```python
from build123d import *

# Parameters (mm, degrees)
BOSS_EXTRUDE1_DEPTH      = 2.5
BOSS_EXTRUDE1_DEPTH_BACK = 2.5
SKETCH1_R                = 18.5
SKETCH1_R_2              = 12.5
SKETCH2_R                = 1.5
CUT_EXTRUDE1_DEPTH       = 10


with BuildPart() as part:
    # Sketch1 → Boss-Extrude1 (new, two sides: drawn at the far end of the back side and taken through both)
    # profile 1 of 2: a face of its own
    with BuildSketch(Plane.XY.offset(-BOSS_EXTRUDE1_DEPTH_BACK)):
        with BuildLine():
            ThreePointArc((18.5, 0), (0, -18.5), (-18.5, 0))
            Line((-18.5, 0), (-18.5, -18.75))
            Line((-18.5, -18.75), (18.5, -18.75))
            Line((18.5, -18.75), (18.5, 0))
        make_face()
    # profile 2 of 2: a face of its own
    with BuildSketch(Plane.XY.offset(-BOSS_EXTRUDE1_DEPTH_BACK)):
        Circle(SKETCH1_R)
        Circle(SKETCH1_R_2, mode=Mode.SUBTRACT)
    extrude(amount=BOSS_EXTRUDE1_DEPTH + BOSS_EXTRUDE1_DEPTH_BACK)

    # Sketch2 → Cut-Extrude1 (cut)
    with BuildSketch(Plane.XZ.offset(18.75)):
        with Locations(Location((-16, 0, 0), (0, 0, 270))):
            Circle(SKETCH2_R)
    cut_extrude1 = extrude(amount=-CUT_EXTRUDE1_DEPTH, mode=Mode.SUBTRACT)

    # Mirror1: Cut-Extrude1 across plane
    add(cut_extrude1.mirror(Plane(origin=(0, 0, 0), x_dir=(0, 0, 1), z_dir=(1, 0, 0))), mode=Mode.SUBTRACT)


solid = part.part
```
Here's how the part is built. I have some questions about the finished solid (model axes, mm). A direction names the side the tool comes from. Round coordinates to 2 decimals unless told otherwise and drop trailing zeros. Write each loop counter-clockwise with the first axis right and the second up, starting at its lowest first coordinate (ties: lowest second). Pieces come first, ordered by that corner, then holes. Notation, with made-up numbers: M 0,-11.5 L 40,-11.5 A26 cw 40,3.5 Z; hole C -9,-0.75 d8. An arc over 180 degrees is marked long. Answer as CSV lines item,"result". Start each with the question number.
1. Suppose I cut it at D-D on y = -14. Write out the boundary of the cut face in (x, z), then the cut area to 3 significant figures.
2. Thinking about a two-plate mould opening in Y: for faces 1 (the cylindrical face through (11.923, 3.755, -0.035)), 2 (the cylindrical face through (-15.55, -13.82, -1.43)), 3 (the flat face through (-16, -8.75, 0)), which applies, released by +Y, released by -Y, zero draft, split by the parting line, or undercut?
3. I'm going to push flat-ended pins straight in: pin 1 Ø1.5 at (x, z) = (13.5, 1) entering from +Y; pin 2 Ø1.8 at (x, z) = (-16, 0) entering from +Y; pin 3 Ø1.5 at (x, z) = (-16, 0) entering from -Y. Where does each tip first touch, or does it pass through?
4. I need wall thicknesses on probe 1 along Z at (x, y) = (16, -11.5); probe 2 along Y at (x, z) = (0, 1.4); probe 3 along X at (y, z) = (-11.5, 0). Which ranges of each line are inside material? Lowest first, please.
5. Suppose I cut it at A-A on x = 0. Write out the boundary of the cut face in (y, z), then the cut area to 4 significant figures.
6. On a 3-axis mill with a long thin cutter (end or side, diameter ignored), from which of +Z, -Z, +X, -X, +Y, -Y can I reach the whole of each face in a straight line? I mean faces 4 (the flat face through (-18.5, -9, 0)), 5 (the flat face through (16, -8.75, 0)). Say none if no direction works.
7. Suppose I cut it at C-C on y = 9.5. Write out the boundary of the cut face in (x, z), then the cut area to 3 significant figures.
8. Suppose I cut it at B-B on z = 0. Write out the boundary of the cut face in (x, y), then the cut area to 3 significant figures.
Check result:
1,outline,"M -18.5,-2.5 L 18.5,-2.5 L 18.5,2.5 L -18.5,2.5 Z; hole C -16,0 d3; hole C 16,0 d3"
1,area,"171 mm2"
2,face 1,"undercut"
2,face 2,"zero draft"
2,face 3,"released by -Y"
3,pin 1,"stops at y = 13.4"
3,pin 2,"stops at y = 10.69"
3,pin 3,"stops at y = -8.75"
4,probe 1,"z = -2.5 to -1.5, 1.5 to 2.5"
4,probe 2,"y = -18.75 to -12.5, 12.5 to 18.5"
4,probe 3,"x = -18.5 to -17.5, -14.5 to -4.9, 4.9 to 14.5, 17.5 to 18.5"
5,outline,"M -18.75,-2.5 L -12.5,-2.5 L -12.5,2.5 L -18.75,2.5 Z; M 12.5,-2.5 L 18.5,-2.5 L 18.5,2.5 L 12.5,2.5 Z"
5,area,"61.25 mm2"
6,face 4,"+Z, -Z, -X, +Y, -Y"
6,face 5,"-Y"
7,outline,"M -15.87,-2.5 L -8.12,-2.5 L -8.12,2.5 L -15.87,2.5 Z; M 8.12,-2.5 L 15.87,-2.5 L 15.87,2.5 L 8.12,2.5 Z"
7,area,"77.5 mm2"
8,outline,"M -18.5,-18.75 L -17.5,-18.75 L -17.5,-8.75 L -14.5,-8.75 L -14.5,-18.75 L 14.5,-18.75 L 14.5,-8.75 L 17.5,-8.75 L 17.5,-18.75 L 18.5,-18.75 L 18.5,0 A18.5 ccw -18.5,0 Z; hole C 0,0 d25"
8,area,"680 mm2"
